```python
from build123d import *

# Parameters (mm, degrees)
SKETCH1_R                = 68.9
BOSS_EXTRUDE1_DEPTH      = 2.3
SKETCH2_R                = 17.75
CUT_EXTRUDE1_DEPTH       = 5.6
CIRPATTERN1_COUNT        = 5
SKETCH3_R                = 72.9
SKETCH3_R_2              = 68.9
BOSS_EXTRUDE2_DEPTH      = 10.9
BOSS_EXTRUDE2_DEPTH_BACK = 9.7
SKETCH4_R                = 11.65
BOSS_EXTRUDE3_DEPTH      = 8
SKETCH6_R                = 1.5
CUT_EXTRUDE2_DEPTH       = 13.6


with BuildPart() as part:
    # Sketch1 → Boss-Extrude1 (new body, symmetric)
    with BuildSketch(Plane.XY):
        Circle(SKETCH1_R)
    extrude(amount=BOSS_EXTRUDE1_DEPTH, both=True)

    # Sketch2 → Cut-Extrude1 (cut, through all)
    with BuildSketch(Plane.XY.offset(2.3)):
        with Locations((0, 39.35)):
            Circle(SKETCH2_R)
    cut_extrude1 = extrude(amount=-CUT_EXTRUDE1_DEPTH, mode=Mode.SUBTRACT)

    # CirPattern1: Cut-Extrude1 ×5 about axis
    cirpattern1_axis = Axis((0, 0, 0), (0, 0, 1))
    for i in range(1, CIRPATTERN1_COUNT):
        add(cut_extrude1.rotate(cirpattern1_axis, i * 360 / CIRPATTERN1_COUNT), mode=Mode.SUBTRACT)

    # Sketch3 → Boss-Extrude2 (add, two sides)
    with BuildSketch(Plane.XY.offset(2.3)) as boss_extrude2_sk:
        Circle(SKETCH3_R)
        Circle(SKETCH3_R_2, mode=Mode.SUBTRACT)
    extrude(amount=BOSS_EXTRUDE2_DEPTH)
    extrude(boss_extrude2_sk.sketch, amount=-BOSS_EXTRUDE2_DEPTH_BACK)

    # Sketch4 → Boss-Extrude3 (add)
    with BuildSketch(Plane(origin=(0, 0, -2.3), x_dir=(-1, 0, 0), z_dir=(0, 0, -1))):
        Circle(SKETCH4_R)
    extrude(amount=BOSS_EXTRUDE3_DEPTH)

    # Sketch6 → Cut-Extrude2 (cut, through all)
    with BuildSketch(Plane.XY.offset(2.3)):
        Circle(SKETCH6_R)
    extrude(amount=-CUT_EXTRUDE2_DEPTH, mode=Mode.SUBTRACT)


solid = part.part
```
Can you work these out from the model? Positions are in its coordinate system, mm. A direction names the side the tool comes from. Give positions to 0.01 mm unless a question says otherwise; leave off trailing zeros. Loops run counter-clockwise (first coordinate to the right, second up) from the corner with the lowest first, then second, coordinate; pieces in that order, holes last. Notation, with made-up numbers: M -14.75,-28.75 L 35.25,-28.75 A23 cw 35.25,8.25 Z; hole C 27.5,48 d10. An arc over 180 degrees is marked long. Use one line per item in the form item = value. Start each with the question number.
(1) I'm going to push flat-ended pins straight in: P1, Ø3.5, axis at x = 0, y = 0, coming from the -Z side; P2, Ø8, axis at y = -43.5, z = 2, coming from the -X side; P3, Ø2, axis at y = -49.5, z = 4.5, coming from the +X side; P4, Ø12, axis at y = 12.5, z = 5.5, coming from the -X side. Where does each tip first touch, or does it pass through?
(2) I want a section at A-A, the plane x = -23.5. Write out the boundary of the cut face in (y, z).
(3) I want a section at B-B, the plane z = -4.75. Write out the boundary of the cut face in (x, y), and give its area (3 significant figures).
(4) Thinking about a two-plate mould opening in Y: for faces 1 (the cylindrical face through (69.534, 21.897, 3.044)), 2 (the flat face through (-2, 0, -10.3)), 3 (the cylindrical face through (2.53, -11.37, -6.24)), which applies, released by +Y, released by -Y, zero draft, split by the parting line, or undercut?
(5) Please list where these lines run through material, in increasing order: line 1 (Y direction, x = 0, z = -6.05); line 2 (X direction, y = -43, z = 1.5); line 3 (Y direction, x = 16, z = -2).
(6) I want a section at C-C, the plane y = 39.35. Write out the boundary of the cut face in (x, z).
(7) I want a section at D-D, the plane y = -29.5. Write out the boundary of the cut face in (x, z).
(8) On a 3-axis mill with a long thin cutter (end or side, diameter ignored), from which of +Z, -Z, +X, -X, +Y, -Y can I reach the whole of each face in a straight line? I mean faces 4 (the flat face through (14, 1, 2.3)), 5 (the cylindrical face through (47.73, -2.29, 0.03)), 6 (the flat face through (14, 1, -2.3)). Say none if no direction works.
Worked out:
q1.P1 = -10.3
q1.P2 = -61.27
q1.P3 = 54.43
q1.P4 = -72.61
q2.outline = M -69.01,-7.4 L -64.77,-7.4 L -64.77,-2.3 L -49.58,-2.3 L -49.58,2.3 L -64.77,2.3 L -64.77,13.2 L -69.01,13.2 Z; M -14.09,-2.3 L 1.15,-2.3 L 1.15,2.3 L -14.09,2.3 Z; M 23.17,-2.3 L 64.77,-2.3 L 64.77,-7.4 L 69.01,-7.4 L 69.01,13.2 L 64.77,13.2 L 64.77,2.3 L 23.17,2.3 Z
q3.outline = C 0,0 d145.8; C 0,0 d23.3; hole C 0,0 d137.8; hole C 0,0 d3
q3.area = 2,200 mm²
q4.face_1 = split by the parting line
q4.face_2 = zero draft
q4.face_3 = undercut
q5.line_1 = -72.9 to -68.9, -11.65 to -1.5, 1.5 to 11.65, 68.9 to 72.9
q5.line_2 = -58.87 to -36.93, -9.33 to 9.33, 36.93 to 58.87
q5.line_3 = -71.12 to -48.09, -15.58 to 31.66, 47.04 to 71.12
q6.outline = M -61.37,-7.4 L -56.56,-7.4 L -56.56,-2.3 L -17.75,-2.3 L -17.75,2.3 L -56.56,2.3 L -56.56,13.2 L -61.37,13.2 Z; M 17.75,-2.3 L 56.56,-2.3 L 56.56,-7.4 L 61.37,-7.4 L 61.37,13.2 L 56.56,13.2 L 56.56,2.3 L 17.75,2.3 Z
q7.outline = M -66.66,-7.4 L -62.27,-7.4 L -62.27,-2.3 L -40.73,-2.3 L -40.73,2.3 L -62.27,2.3 L -62.27,13.2 L -66.66,13.2 Z; M -5.53,-2.3 L 5.53,-2.3 L 5.53,2.3 L -5.53,2.3 Z; M 40.73,-2.3 L 62.27,-2.3 L 62.27,-7.4 L 66.66,-7.4 L 66.66,13.2 L 62.27,13.2 L 62.27,2.3 L 40.73,2.3 Z
q8.face_4 = +Z
q8.face_5 = +Z, -Z
q8.face_6 = -Z
